Autodesk Inventor part; units mm, degrees
ref_plane "YZ Plane" through (0, 0, 0) normal (1, 0, 0) x (0, 1, 0)
ref_plane "XZ Plane" through (0, 0, 0) normal (0, 1, 0) x (-1, 0, 0)
ref_plane "XY Plane" through (0, 0, 0) normal (0, 0, 1) x (1, 0, 0)
sketch "Sketch_3" plane through (0, 0, 0) normal (0, 0, 1) x (1, 0, 0)
  line L0 (63, 0) -> (0, 0)
  line L1 (0, 0) -> (0, 5.5)
  line L2 (0, 5.5) -> (0.5, 6)
  line L3 (0.5, 6) -> (62.5, 6)
  line L4 (62.5, 6) -> (63, 5.5)
  line L5 (63, 5.5) -> (63, 0)
  line L6 (63, 0) -> (0, 0)
revolve "Revolution1" add sketch "Sketch_3" angle 360 about axis through (63, 0, 0) along (1, 0, 0)
sketch "Sketch_10" plane through (22, 0, 0) normal (1, 0, 0) x (0, 0, -1)
  line L0 (-12, 12) -> (-12, -12)
  line L1 (-12, -12) -> (-5, -12)
  line L2 (-5, -12) -> (-5, 5)
  line L3 (-5, 5) -> (12, 5)
  line L4 (12, 5) -> (12, 12)
  line L5 (12, 12) -> (-12, 12)
extrude "Extrusion1" cut sketch "Sketch_10" along normal blind 6
properties part number "PSSFG12-63-RC22"
For this review, take the finished solid that the model builds, in its own axes (mm). A direction names the side the tool comes from. Give positions to 0.01 mm unless a question says otherwise; leave off trailing zeros. Order: outer loops, then holes, each group sorted by start corner. A loop starts at its lowest first (then second) coordinate and runs counter-clockwise, first axis right, second up.
1) The part is to be moulded in two halves that separate along X. For faces 4 (the face through (22, 5.4, 0)), 5 (the face through (63, 0, 0)), 6 (the face through (0, 0, 0)), 7 (the face through (25, 5, 0)), say which applies: released by +X, released by -X, zero draft, split by the parting line, or undercut.
2) Take a section at A-A (x = 7.5). Give the boundary of the cut face in (y, z).
3) Insertion check: pin 1 (3 mm diameter, centred on x = 11.5, z = -4.5, fed in from -Y); pin 2 (1 mm diameter, centred on x = 40.5, z = 3.5, fed in from +Y); pin 3 (4 mm diameter, centred on x = 17, z = 3, fed in from +Y). Each pin has a flat end and moves straight along its axis. Give the tip position at first contact, or say it passes through.
4) For faces 1 (the face through (25, 0, 5)), 2 (the face through (31.93, -4.76, -3.65)), 3 (the face through (28, 5.4, 0)), list the 3-axis set-ups (+Z, -Z, +X, -X, +Y, -Y) from which the entire face can be reached by the end or side of a thin tool; tool diameter is ignored.
5) Wall thickness on line 1 (Y direction, x = 54.5, z = 5); line 2 (Z direction, x = 51, y = -0.25); line 3 (Y direction, x = 9.5, z = 3.5): over which ranges is each line inside the solid? List them lowest first.
Derived:
1. face 4: undercut
1. face 5: released by +X
1. face 6: released by -X
1. face 7: undercut
2. outline: circle Ø12 at (0, 0)
3. pin 1: stops at y = -5.2
3. pin 2: stops at y = 5.2
3. pin 3: stops at y = 5.92
4. face 1: +Z, +Y, -Y
4. face 2: +X, -X
4. face 3: +Z, -Z, +Y
5. line 1: y = -3.32 to 3.32
5. line 2: z = -5.99 to 5.99
5. line 3: y = -4.87 to 4.87
